Work out the finished part from the listing and answer in its coordinate system (mm). Face numbers are marked on the shaded views. A direction names the side the tool comes from. Give positions to 0.01 mm unless a question says otherwise; leave off trailing zeros. Loops run counter-clockwise (first coordinate to the right, second up) from the corner with the lowest first, then second, coordinate; pieces in that order, holes last. Notation, with made-up numbers: M 55.5,15 L 67.5,15 A3 ccw 67.5,20 Z; hole C -32.5,-28 d6. An arc over 180 degrees is marked long. Use a Markdown table: item, result.
```python
from build123d import *

# Parameters (mm, degrees)
CYLINDER_R        = 13
CYLINDER_DEPTH    = 45
CYLINDER001_R     = 14
CYLINDER001_DEPTH = 10
CYLINDER002_R     = 15
CYLINDER002_DEPTH = 80
CHAMFER_SIZE      = 2
FILLET_R          = 10
BOX_W             = 80
BOX_H             = 80
BOX_DEPTH         = 15


with BuildPart() as part:
    # Cylinder → Cylinder (join)
    with BuildSketch(Plane.XY):
        Circle(CYLINDER_R)
    extrude(amount=CYLINDER_DEPTH)

    # Cylinder001 → Cylinder001 (join)
    with BuildSketch(Plane.XY.offset(45)):
        Circle(CYLINDER001_R)
    extrude(amount=CYLINDER001_DEPTH)

    # Cylinder002 → Cylinder002 (join)
    with BuildSketch(Plane(origin=(-40, 0, 60), x_dir=(0, 1, 0), z_dir=(1, 0, 0))):
        Circle(CYLINDER002_R)
    extrude(amount=CYLINDER002_DEPTH)

    # Chamfer
    chamfer_edges = [part.edges().sort_by_distance(p)[0] for p in [
        (-13, 0, 0),
    ]]
    chamfer(chamfer_edges, length=CHAMFER_SIZE)

    # Fillet
    fillet_edges = [part.edges().sort_by_distance(p)[0] for p in [
        (40, -15, 60),
        (-40, -15, 60),
    ]]
    fillet(fillet_edges, radius=FILLET_R)

    # Box → Box (cut)
    with BuildSketch(Plane(origin=(-40, 15, 0), x_dir=(1, 0, 0), z_dir=(0, -1, 0))):
        with Locations((40, 40)):
            Rectangle(BOX_W, BOX_H)
    extrude(amount=BOX_DEPTH, mode=Mode.SUBTRACT)


solid = part.part
```
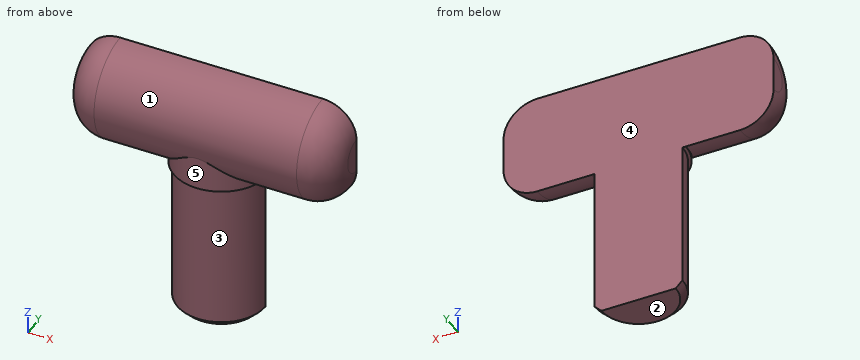
(1) A cutting plane is placed at C-C (x = 17). Write down the section's boundary in (y, z), and give its area (3 significant figures).
Entries:
| item | result |
|---|---|
| outline | M 0,45 L 0,75 A15 ccw Z |
| area | 353 mm² |
(2) Consider probe 1 along Z at (x, y) = (-7, -0.75); probe 2 along Z at (x, y) = (-3, -7.25); probe 3 along X at (y, z) = (-9.25, 27). Determine where each line is inside the solid, lowest interval first. Write a range as [from, to].
Entries:
| item | result |
|---|---|
| probe 1 | z = [0, 74.98] |
| probe 2 | z = [0, 73.13] |
| probe 3 | x = [-9.13, 9.13] |
(3) A cutting plane is placed at B-B (z = 9). Write down the section's boundary in (x, y).
Entries:
| item | result |
|---|---|
| outline | M -13,0 A13 ccw 13,0 Z |
(4) The mould has two halves that part along Z. Classify the marked faces 1, 2 and 3: released by +Z, released by -Z, zero draft, split by the parting line, or undercut.
Entries:
| item | result |
|---|---|
| face 1 | split by the parting line |
| face 2 | released by -Z |
| face 3 | zero draft |
(5) Which of the six approach directions +Z, -Z, +X, -X, +Y, -Y give full straight-line access (tool end or side, diameter ignored) to the marked faces 4 and 5?
Entries:
| item | result |
|---|---|
| face 4 | +Z, -Z, +X, -X, +Y |
| face 5 | -Z, -Y |
(6) A cutting plane is placed at A-A (x = 0). Write down the section's boundary in (y, z), and give its area (3 significant figures).
Entries:
| item | result |
|---|---|
| outline | M -14,45 L -13,45 L -13,2 L -11,0 L 0,0 L 0,75 A15 ccw -14,54.61 Z |
| area | 973 mm² |
(7) Given P1, Ø5, axis at x = -30, y = -8.5, coming from the -Z side; P2, Ø5, axis at x = -24, z = 57.5, coming from the -Y side; P3, Ø5, axis at x = -11, y = -5, coming from the +Z side; P4, Ø5, axis at y = -10.5, z = 52, coming from the -X side, each flat-ended and moving along its own axis, determine where each tip first touches the part or whether it passes through.
Entries:
| item | result |
|---|---|
| P1 | stops at z = 46.25 |
| P2 | stops at y = -15 |
| P3 | stops at z = 74.79 |
| P4 | stops at x = -38.22 |
